from build123d import *

# Parameters (mm, degrees)
F0_W     = 63.5
F0_H     = 31.75
F1_DEPTH = 25.4
F2_W     = 57.15
F2_H     = 25.4
F3_DEPTH = 19.05
F4_R     = 7.62
F5_SIZE  = 1.27


with BuildPart() as f1:
    # F0 (on Top) → F1 (new body)
    with BuildSketch(Plane.XY):
        with Locations((31.75, 15.875)):
            Rectangle(F0_W, F0_H)
    extrude(amount=F1_DEPTH)

    # F2 (on face) → F3 (cut)
    with BuildSketch(Plane.XY.offset(25.4)):
        with Locations((28.575, 12.7)):
            Rectangle(F2_W, F2_H)
    extrude(amount=-F3_DEPTH, mode=Mode.SUBTRACT)

    # F4
    f4_edges = [f1.edges().sort_by_distance(p)[0] for p in [
        (28.575, 25.4, 6.35),
        (57.15, 12.7, 6.35),
        (57.15, 25.4, 15.875),
    ]]
    fillet(f4_edges, radius=F4_R)

    # F5
    f5_edges = [f1.edges().sort_by_distance(p)[0] for p in [
        (63.5, 15.875, 25.4),
        (31.75, 31.75, 25.4),
    ]]
    chamfer(f5_edges, length=F5_SIZE)


solid = f1.part
Design review of the part built by this model. Coordinates are the model's own, in mm. A direction names the side the tool comes from. Coordinates: 2 decimals unless noted, no trailing zeros. Loops run counter-clockwise (first coordinate to the right, second up) from the corner with the lowest first, then second, coordinate; pieces in that order, holes last. Notation, with made-up numbers: M -10,67 L 7,67 A20 cw 7,95 Z; hole C 30,-25 d4. An arc over 180 degrees is marked long. Answer as CSV lines item,"result".
Item 1: Add section C-C on x = 24. State the section outline as (y, z) points.
Answer list:
outline,"M 0,0 L 31.75,0 L 31.75,24.13 L 30.48,25.4 L 25.4,25.4 L 25.4,13.97 A7.62 cw 17.78,6.35 L 0,6.35 Z"
Item 2: For probe 1 along X at (y, z) = (3, 20.75); probe 2 along Y at (x, z) = (47, 22.5); probe 3 along Z at (x, y) = (15, 17.5), list the stretches that pass through material, from the lowest coordinate up.
Answer list:
probe 1,"57.15 to 63.5"
probe 2,"25.4 to 31.75"
probe 3,"0 to 6.35"
Item 3: For P1, Ø9, axis at x = 23, z = 18, coming from the -Y side; P2, Ø1.5, axis at x = 56.5, z = 11, coming from the -Y side; P3, Ø2, axis at x = 53.5, z = 16, coming from the -Y side; P4, Ø12.5, axis at y = 4.5, z = 20, coming from the -X side, all flat-tipped, find the tip position at first contact; note any pin that passes through.
Answer list:
P1,"y = 25.39"
P2,"y = 0"
P3,"y = 23.56"
P4,"x = 57.15"
Item 4: Add section D-D on z = 7.5. State the section outline as (x, y) points.
Answer list:
outline,"M 0,21.81 L 49.53,21.81 A4.03 cw 53.56,17.78 L 53.56,0 L 63.5,0 L 63.5,31.75 L 0,31.75 Z"
Item 5: Add section A-A on y = 6. State the section outline as (x, z) points, plus the area to 3 significant figures.
Answer list:
outline,"M 0,0 L 63.5,0 L 63.5,24.13 L 62.23,25.4 L 57.15,25.4 L 57.15,13.97 A7.62 cw 49.53,6.35 L 0,6.35 Z"
area,"536 mm²"
Item 6: Add section B-B on z = 19.25. State the section outline as (x, y) points.
Answer list:
outline,"M 0,25.4 L 49.53,25.4 A7.62 cw 57.15,17.78 L 57.15,0 L 63.5,0 L 63.5,31.75 L 0,31.75 Z"
Item 7: Machinability: for faces 1 (the face through (24, 9, 6.35)), 2 (the face through (0, 23, 7)), which of the approach directions +Z, -Z, +X, -X, +Y, -Y give a long, thin tool a straight path to every point of the face, cutting with its end or side? Answer none if there is none.
Answer list:
face 1,"+Z, -X, -Y"
face 2,"+Z, -Z, -X, +Y, -Y"
